For this review, take the finished solid that the model builds, in its own axes (mm). Coordinates: 2 decimals unless noted, no trailing zeros. Loops run counter-clockwise (first coordinate to the right, second up) from the corner with the lowest first, then second, coordinate; pieces in that order, holes last.
1. Take a section at D-D, the plane y = 215. State the section outline as (x, z) points.
2. To check wall thickness, follow probe 1 along Y at (x, z) = (0, -1.3); probe 2 along X at (y, z) = (247, -1.05); probe 3 along X at (y, z) = (25, -0.25). State the ranges of each line that lie inside material, in increasing order.
3. Clearance check with flat-ended pins moving along their axes: P1, Ø1.6, axis at y = 115.5, z = -2.5, coming from the +X side; P2, Ø3, axis at y = 55, z = -3, coming from the +X side; P3, Ø3, axis at x = 21, y = 132, coming from the +Z side; P4, Ø3, axis at x = -44.5, z = -4.5, coming from the +Y side. State where each tip first meets the part, or that it passes through.
4. Take a section at A-A, the plane z = -3.05. State the section outline as (x, y) points, then the cut area to 3 significant figures.
5. Take a section at B-B, the plane y = 62.5. State the section outline as (x, z) points, then the cut area to 3 significant figures.
6. Take a section at C-C, the plane y = 121. State the section outline as (x, z) points, then the cut area to 3 significant figures.
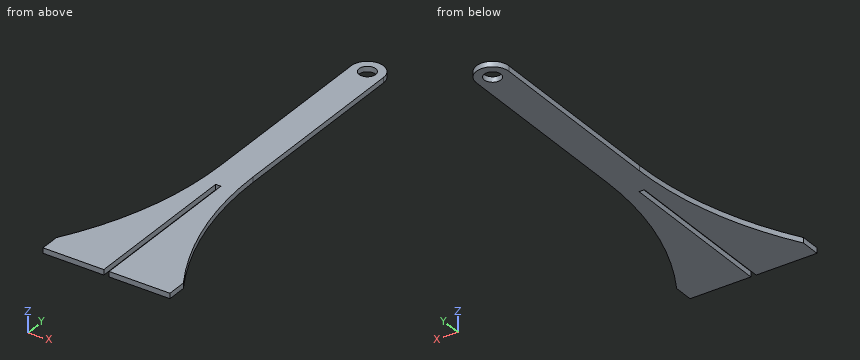
```python
from build123d import *

# Parameters (mm, degrees)
SKETCH2_R           = 8.5
BOSS_EXTRUDE1_DEPTH = 5.4
CAVITY1_START       = -2.7
CAVITY1_OUTLINE_W   = 167.1
CAVITY1_OUTLINE_H   = 5.4
CAVITY1_DEPTH       = 5.4


# Read off the part's stored shape, not the designer's step: Cavity1
with BuildPart() as part:
    # Sketch2 → Boss-Extrude1 (new body)
    with BuildSketch(Plane.XY):
        with BuildLine():
            Line((-65, 0), (65, 0))
            Line((65, 0), (65, 20))
            ThreePointArc((65, 20), (28.922939589, 104.215144435), (16.6, 195))
            Line((16.6, 195), (16.6, 390))
            ThreePointArc((16.6, 390), (0, 406.6), (-16.6, 390))
            Line((-16.6, 390), (-16.6, 195))
            ThreePointArc((-16.6, 195), (-28.922939589, 104.215144435), (-65, 20))
            Line((-65, 20), (-65, 0))
        make_face()
        with Locations((0, 390)):
            Circle(SKETCH2_R, mode=Mode.SUBTRACT)
    extrude(amount=-BOSS_EXTRUDE1_DEPTH)

    # Cavity1 outline → Cavity1 (cut)
    with BuildSketch(Plane.YZ.offset(CAVITY1_START)):
        with Locations((83.55, -2.7)):
            Rectangle(CAVITY1_OUTLINE_W, CAVITY1_OUTLINE_H)
    extrude(amount=CAVITY1_DEPTH, mode=Mode.SUBTRACT)


solid = part.part
```
Results list:
1. outline: (-16.6, -5.4) - (16.6, -5.4) - (16.6, 0) - (-16.6, 0) - close
2. probe 1: y = 167.1 to 381.5, 398.5 to 406.6
2. probe 2: x = -16.6 to 16.6
2. probe 3: x = -62.06 to -2.7, 2.7 to 62.06
3. P1: stops at x = 26.2
3. P2: stops at x = 47.39
3. P3: stops at z = 0
3. P4: stops at y = 63.53
4. outline: (-65, 0) - (-2.7, 0) - (-2.7, 167.1) - (2.7, 167.1) - (2.7, 0) - (65, 0) - (65, 20) arc R340.57 cw to (16.6, 195) - (16.6, 390) arc R16.6 ccw to (-16.6, 390) - (-16.6, 195) arc R340.57 cw to (-65, 20) - close; hole circle Ø17 at (0, 390)
4. area: 19,700 mm2
5. outline: (-43.43, -5.4) - (-2.7, -5.4) - (-2.7, 0) - (-43.43, 0) - close; (2.7, -5.4) - (43.43, -5.4) - (43.43, 0) - (2.7, 0) - close
5. area: 440 mm2
6. outline: (-24.74, -5.4) - (-2.7, -5.4) - (-2.7, 0) - (-24.74, 0) - close; (2.7, -5.4) - (24.74, -5.4) - (24.74, 0) - (2.7, 0) - close
6. area: 238 mm2
